Check sheet for the modelled part. Datum: model origin and axes. Units: mm. Round coordinates to 2 decimals unless told otherwise and drop trailing zeros. Order: outer loops, then holes, each group sorted by start corner. A loop starts at its lowest first (then second) coordinate and runs counter-clockwise, first axis right, second up.
Q1. Scan lines: probe 1 along X at (y, z) = (0.25, -19.5); probe 2 along X at (y, z) = (1.4, -37.5); probe 3 along X at (y, z) = (2.4, -53). Record each from-to range of solid material in increasing order.
Q2. Cross-section at C-C on z = -25.5. Record the cut outline in (x, y).
Q3. Cross-section at A-A on y = 1.35. Record the cut outline in (x, z), then the cut area to 3 significant figures.
Q4. Depth check by flat-ended pin: P1, Ø0.8, axis at y = 1, z = -24, coming from the -X side; P2, Ø1.2, axis at y = 1, z = -24, coming from the +X side. Enter the tip coordinate at first touch or a pass-through.
Q5. Cross-section at B-B on x = 5. Record the cut outline in (y, z), then the cut area to 3 significant figures.
Q6. Cross-section at D-D on x = -3. Record the cut outline in (y, z).
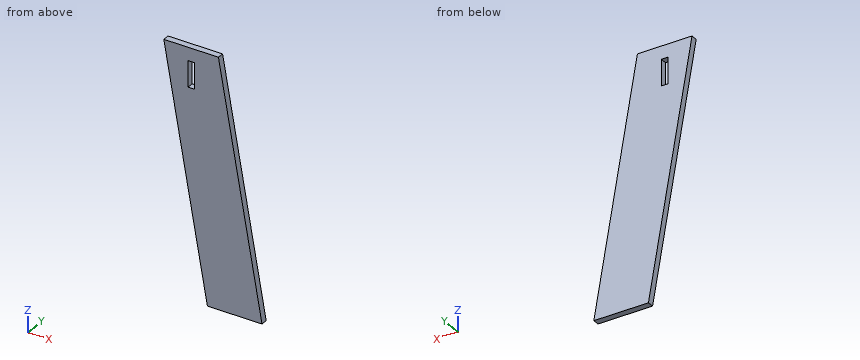
Autodesk Inventor part; units mm, degrees
ref_plane "YZ Plane" through (0, 0, 0) normal (1, 0, 0) x (0, 1, 0)
ref_plane "XZ Plane" through (0, 0, 0) normal (0, 1, 0) x (-1, 0, 0)
ref_plane "XY Plane" through (0, 0, 0) normal (0, 0, 1) x (1, 0, 0)
sketch "スケッチ1" plane through (0, 0, 0) normal (0, 1, 0) x (-1, 0, 0)
  circle A0 centre (0, 0) radius 11
  line L0 (11, 10) -> (-11, 10)
  line L1 (-11, 10) -> (-11, -10)
  line L2 (-11, -10) -> (11, -10)
  line L3 (11, -10) -> (11, 10)
  line L4 (11, -10) -> (-11, -10)
  line L5 (-11, -10) -> (-11, -110)
  line L6 (-11, -110) -> (11, -110) construction
  line L7 (11, -110) -> (11, -10) construction
  arc A1 (-34.6127, -115.6757) -> (-13.3752, -120) centre (0, 0) ccw
  circle A2 centre (22, 0) radius 11
  circle A3 centre (-22, 0) radius 11
  line L8 (46.542, 0) -> (-48.2519, 0)
  line L9 (0, 0) -> (-13.7873, 2.4311)
  line L10 (-13.7873, 2.4311) -> (-34.6127, -115.6757)
  line L11 (22, 0) -> (8.2127, 2.4311)
  line L12 (8.2127, 2.4311) -> (-13.3752, -120)
  line L13 (8.2127, 2.4311) -> (8.9192, 6.438)
  line L14 (-13.7873, 2.4311) -> (-7.33, 8.2019)
  point P0 (11, 0)
  point P1 (11, 0)
  point P2 (4.5826, 10)
  point P3 (-4.5826, 10)
  point P4 (-11, 0)
  point P5 (-11, 0)
  point P6 (-11, 0)
  point P7 (4.5826, -10)
  point P8 (11, 0)
  point P9 (-11, 0)
  point P10 (-4.5826, -10)
  point P11 (4.5826, -10)
  point P12 (-4.5826, -10)
  point P13 (6.1794, -9.1003)
  point P14 (7.784, 0)
  point P15 (10.822, 1.971)
  point P16 (-14.216, 0)
  point P17 (11, 1.9396)
  dimension "d0" = 22
  dimension "d1" = 20
  dimension "d2" = 100
  dimension "d13" = 10
  dimension "d14" = 14
  dimension "d15" = 10
extrude "押し出し1" add sketch "スケッチ1" along normal blind 2.5 contours L12 L2 A0 | A0 L2 L8 L12 | L8 L9 A0 L0 L13 L12 | L2 L12 L5 A0 | A0 L2 | L8 A0 L9 | L2 L1 A0 | L12 A1 L10 A3 L1 L5 | L1 L9 A0 | A3 L9 L1 | L8 L10 L9 A3 | A3 L10 L8 | L9 L1 L14 A0 | L9 A3 L14 L1 | L9 L14 A3 picked at (-14.6149, -5.4805)
sketch "スケッチ2" plane through (0, 2.5, 0) normal (0, 1, 0) x (1, 0, 0)
  line L0 (33.6474, 115.9601) -> (12.5819, -3.5083)
  line L1 (13.7873, -2.4311) -> (34.6127, 115.6757)
  arc A0 (34.6127, 115.6757) -> (13.3752, 120) centre (0, 0) ccw
  line L2 (7.33, -8.2019) -> (13.7873, -2.4311)
  dimension "d16" = 1
extrude "押し出し2" cut sketch "スケッチ2" against normal through all
sketch "スケッチ3" plane through (0, 2.5, 0) normal (0, 1, 0) x (1, 0, 0)
  line L0 (-11, 14) -> (-4, 14)
  line L1 (-4, 14) -> (16.0696, 14)
  line L2 (12.5819, -3.5083) -> (33.6474, 115.9601)
  arc A0 (33.6474, 115.9601) -> (13.3752, 120) centre (0, 0) ccw
  line L3 (13.3752, 120) -> (-8.9192, -6.438)
  arc A1 (-8.9192, -6.438) -> (-4.5826, -10) centre (0, 0) ccw
  line L4 (-4.5826, -10) -> (4.5826, -10)
  arc A2 (4.5826, -10) -> (7.33, -8.2019) centre (0, 0) ccw
  line L5 (7.33, -8.2019) -> (12.5819, -3.5083)
  point P0 (15.6691, 14)
  point P1 (-5.3154, 14)
extrude "押し出し3" cut sketch "スケッチ3" against normal through all contours L0 L1 L2 L5 A2 L4 A1 L3
sketch "スケッチ4" plane through (0, 2.5, 0) normal (0, 1, 0) x (1, 0, 0)
  line L0 (6.5, 29) -> (6.5, 19)
  line L1 (4, 19) -> (4, 29)
  line L2 (4, 29) -> (6.5, 29)
  line L3 (6.5, 19) -> (4, 19)
  point P0 (0, 0)
extrude "押し出し4" cut sketch "スケッチ4" against normal through all
sketch "スケッチ5" plane through (0, 2.5, 0) normal (0, 1, 0) x (1, 0, 0)
  line L0 (11, 109) -> (-11, 109)
  line L1 (11, 109) -> (32.4202, 109)
  line L2 (33.6474, 115.9601) -> (15.6691, 14)
  line L3 (6.5, 19) -> (4, 19)
  line L4 (4, 19) -> (4, 29)
  line L5 (4, 29) -> (6.5, 29)
  line L6 (6.5, 29) -> (6.5, 19)
  line L7 (-5.3154, 14) -> (15.6691, 14)
  line L8 (15.6691, 14) -> (33.6474, 115.9601)
  arc A0 (33.6474, 115.9601) -> (13.3752, 120) centre (0, 0) ccw
  line L9 (13.3752, 120) -> (-5.3154, 14)
  point P0 (11.4356, 109)
extrude "押し出し5" cut sketch "スケッチ5" against normal through all contours L9 A0 L2 L1
properties part number "dish_under" material "木材 (カエデ材)"
Results found:
1. probe 1: x = -4.35 to 4, 6.5 to 16.64
1. probe 2: x = -1.17 to 19.81
1. probe 3: x = 1.56 to 22.55
2. outline: (-3.29, 0) - (4, 0) - (4, 2.5) - (-3.29, 2.5) - close; (6.5, 0) - (17.7, 0) - (17.7, 2.5) - (6.5, 2.5) - close
3. outline: (-5.32, -14) - (11.44, -109) - (32.42, -109) - (15.67, -14) - close; hole (4, -29) - (6.5, -29) - (6.5, -19) - (4, -19) - close
3. area: 1,970 mm2
4. P1: stops at x = -3.62
4. P2: stops at x = 17.54
5. outline: (0, -72.5) - (2.5, -72.5) - (2.5, -29) - (0, -29) - close; (0, -19) - (2.5, -19) - (2.5, -14) - (0, -14) - close
5. area: 121 mm2
6. outline: (0, -27.13) - (2.5, -27.13) - (2.5, -14) - (0, -14) - close
